```python
from build123d import *

# Parameters (mm, degrees)
CUT_EXTRUDE1_START  = -19
SKETCH3_W           = 5
SKETCH3_H           = 8
CUT_EXTRUDE1_DEPTH  = 40
SKETCH4_R           = 12.5
SKETCH4_R_2         = 9.5
CUT_EXTRUDE2_DEPTH  = 1.2
SKETCH5_R           = 8.5
BOSS_EXTRUDE1_DEPTH = 50
SKETCH8_W           = 5
SKETCH8_H           = 3
CUT_EXTRUDE3_DEPTH  = 15
SKETCH9_R           = 8.5
BOSS_EXTRUDE2_DEPTH = 5
SKETCH10_R          = 10.1
SKETCH10_R_2        = 8.1
CUT_EXTRUDE4_DEPTH  = 1
CUT_EXTRUDE5_START  = -1
SKETCH11_R          = 10.1
SKETCH11_R_2        = 8.1
CUT_EXTRUDE5_DEPTH  = 1


with BuildPart() as part:
    # Sketch2 → Revolve1 (revolve)
    with BuildSketch(Plane(origin=(0, 0, 0), x_dir=(0, 0, -1), z_dir=(1, 0, 0)), mode=Mode.PRIVATE) as revolve1_sk:
        Polygon((0, 0), (0, 8.5), (14, 8.5), (14, 12), (19, 12), (19, 10), (98, 10), (98, 8.5), (112, 8.5), (112, 0), align=None)
    revolve(revolve1_sk.sketch.rotate(Axis((0, 0, 0), (0, 0, -1)), 90), axis=Axis((0, 0, 0), (0, 0, -1)))

    # Sketch3 → Cut-Extrude1 (cut)
    with BuildSketch(Plane.XY.offset(CUT_EXTRUDE1_START)):
        with Locations((0, 12)):
            Rectangle(SKETCH3_W, SKETCH3_H)
    extrude(amount=-CUT_EXTRUDE1_DEPTH, mode=Mode.SUBTRACT)

    # Sketch4 → Cut-Extrude2 (cut)
    with BuildSketch(Plane.XY.offset(-59)):
        Circle(SKETCH4_R)
        Circle(SKETCH4_R_2, mode=Mode.SUBTRACT)
    extrude(amount=-CUT_EXTRUDE2_DEPTH, mode=Mode.SUBTRACT)

    # Sketch5 → Boss-Extrude1 (add)
    with BuildSketch(Plane.XY):
        Circle(SKETCH5_R)
    extrude(amount=BOSS_EXTRUDE1_DEPTH)

    # Sketch8 → Cut-Extrude3 (cut)
    with BuildSketch(Plane.XY.offset(50)):
        with Locations((0, 7)):
            Rectangle(SKETCH8_W, SKETCH8_H)
    extrude(amount=-CUT_EXTRUDE3_DEPTH, mode=Mode.SUBTRACT)

    # Sketch9 → Boss-Extrude2 (add)
    with BuildSketch(Plane.XY.offset(50)):
        Circle(SKETCH9_R)
    extrude(amount=BOSS_EXTRUDE2_DEPTH)

    # Sketch10 → Cut-Extrude4 (cut)
    with BuildSketch(Plane(origin=(0, 0, 50), x_dir=(-1, 0, 0), z_dir=(0, 0, -1))):
        Circle(SKETCH10_R)
        Circle(SKETCH10_R_2, mode=Mode.SUBTRACT)
    extrude(amount=-CUT_EXTRUDE4_DEPTH, mode=Mode.SUBTRACT)

    # Sketch11 → Cut-Extrude5 (cut)
    with BuildSketch(Plane.XY.offset(35).offset(CUT_EXTRUDE5_START)):
        Circle(SKETCH11_R)
        Circle(SKETCH11_R_2, mode=Mode.SUBTRACT)
    extrude(amount=CUT_EXTRUDE5_DEPTH, mode=Mode.SUBTRACT)


solid = part.part
```
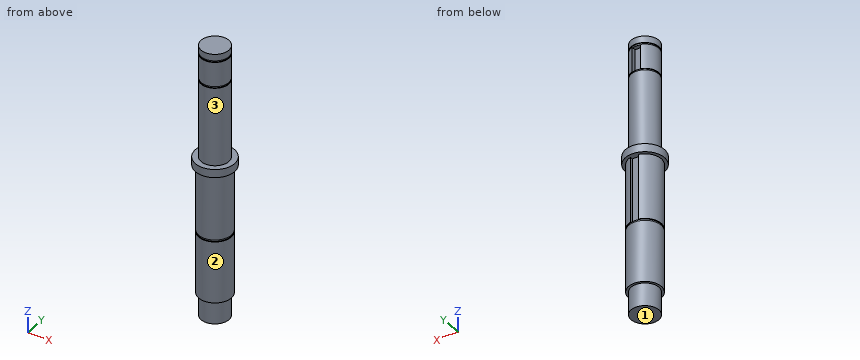
Design review of the part built by this model. Coordinates are the model's own, in mm. Face numbers are marked on the shaded views. A direction names the side the tool comes from. Coordinates: 2 decimals unless noted, no trailing zeros. Loops run counter-clockwise (first coordinate to the right, second up) from the corner with the lowest first, then second, coordinate; pieces in that order, holes last. Notation, with made-up numbers: (10, 24) - (30, 24) arc R12 ccw to (30, 31) - close; hole circle Ø3 at (33.5, 35.25). An arc over 180 degrees is marked (long way). Use CSV: the item, a comma, the result in double quotes. Start each with the question number.
1) Tool access review of the marked faces 1, 2 and 3: name each direction out of +Z, -Z, +X, -X, +Y, -Y from which nothing blocks a thin tool from reaching the whole face with its end or side.
2) For pin 1 Ø5 at (x, z) = (-9.5, -35.5) entering from +Y; pin 2 Ø0.8 at (y, z) = (8.5, -38.5) entering from -X; pin 3 Ø0.8 at (y, z) = (8.5, -29.5) entering from +X, all flat-tipped, find the tip position at first contact; note any pin that passes through.
3) Consider section C-C on z = -27.5. Write out the cut boundary in (x, y), then the cut area to 3 significant figures.
4) Consider section A-A on z = -78. Write out the cut boundary in (x, y), then the cut area to 3 significant figures.
5) Wall thickness on L1, parallel to Z at x = -1.75, y = 8.25; L2, parallel to Z at x = -6.5, y = -6.25; L3, parallel to Z at x = 10, y = -3: over which ranges is each line inside the solid? List them lowest first. Write a range as from..to.
6) Consider section B-B on z = -100. Write out the cut boundary in (x, y).
Geometry says:
1,face 1,"-Z, +X, -X, +Y, -Y"
1,face 2,"-Z"
1,face 3,"+Z"
2,pin 1,"y = 7.14"
2,pin 2,"x = -5.86"
2,pin 3,"x = 5.86"
3,outline,"(-2.5, 8) - (-2.5, 9.68) arc R10 ccw (long way) to (2.5, 9.68) - (2.5, 8) - close"
3,area,"305 mm^2"
4,outline,"circle Ø20 at (0, 0)"
4,area,"314 mm^2"
5,L1,"-112..-59, -19..34, 51..55"
5,L2,"-98..-14"
5,L3,"-19..-14"
6,outline,"circle Ø17 at (0, 0)"
